Could you check a few things on this model? Use its own coordinates, in mm. A direction names the side the tool comes from. Round coordinates to 2 decimals unless told otherwise and drop trailing zeros. Write each loop counter-clockwise with the first axis right and the second up, starting at its lowest first coordinate (ties: lowest second). Pieces come first, ordered by that corner, then holes. Notation, with made-up numbers: (60, 31.5) -> (91, 31.5) arc R32 cw to (91, 68.5) -> close; hole circle Ø8 at (45.25, 64). An arc over 180 degrees is marked (long way). Answer in a Markdown table with one row per item.
from build123d import *

# Parameters (mm, degrees)
SKETCH_W      = 320
SKETCH_H      = 350
PAD_DEPTH     = 590
POCKET_DEPTH  = 50
SKETCH002_W   = 312.833359
SKETCH002_H   = 173.796318
SKETCH002_W_2 = 309.6734
SKETCH002_H_2 = 165.896453
PAD001_DEPTH  = 10
SKETCH003_W   = 329.541511
SKETCH003_H   = 368.861823
PAD002_DEPTH  = 50


with BuildPart() as part:
    # Sketch → Pad (new body)
    with BuildSketch(Plane.XZ):
        with Locations((160, 175)):
            Rectangle(SKETCH_W, SKETCH_H)
    extrude(amount=PAD_DEPTH)

    # Sketch001 (on Face6 of Pad) → Pocket (cut)
    with BuildSketch(Plane.XZ.offset(590)):
        Polygon((-35.069702, 294.049438), (-35.069702, 61.386997), (59.508472, 61.386997), (59.508472, -35.082802), (254.339645, -35.082802), (254.339645, 61.386997), (365.941986, 61.386997), (365.941986, 294.049438), (254.339645, 294.049438), (254.339645, 365.928894), (59.508472, 365.928894), (59.508472, 294.049438), align=None)
    extrude(amount=-POCKET_DEPTH, mode=Mode.SUBTRACT)

    # Sketch002 (on Face9 of Pocket) → Pad001 (join)
    with BuildSketch(Plane(origin=(0, 0, 0), x_dir=(0, 0, -1), z_dir=(-1, 0, 0))):
        with Locations((-177.158851, 160.656223)):
            Rectangle(SKETCH002_W, SKETCH002_H)
        with Locations((-177.158844, 363.681931)):
            Rectangle(SKETCH002_W_2, SKETCH002_H_2)
    extrude(amount=PAD001_DEPTH)

    # Sketch003 (on Face2 of Pad001) → Pad002 (join)
    with BuildSketch(Plane(origin=(0, 0, 0), x_dir=(1, 0, 0), z_dir=(0, 1, 0))):
        with Locations((159.986142, -175.059994)):
            Rectangle(SKETCH003_W, SKETCH003_H)
    extrude(amount=-PAD002_DEPTH)


solid = part.part
1) For pin 1 (1.5 mm diameter, centred on y = -383, z = 81.5, fed in from +X); pin 2 (25 mm diameter, centred on y = -36, z = 192, fed in from -X); pin 3 (8 mm diameter, centred on x = -5.5, y = -182, fed in from -Z), each with a flat end and sliding along its axis, tell me the tip position at first contact or that it passes through.
Findings:
| item | result |
|---|---|
| pin 1 | stops at x = 320 |
| pin 2 | stops at x = -4.78 |
| pin 3 | stops at z = 20.74 |
2) Please list where these lines run through material, in increasing order: line 1 (X direction, y = -143, z = 146); line 2 (Y direction, x = 159, z = 128); line 3 (Z direction, x = 134.5, y = -183).
Findings:
| item | result |
|---|---|
| line 1 | x = -10 to 320 |
| line 2 | y = -540 to 0 |
| line 3 | z = 0 to 350 |
3) Imagine slicing it at C-C, the plane x = 34. Please give me the cut outline in (y, z), plus the area to 3 significant figures.
Findings:
| item | result |
|---|---|
| outline | (-590, 0) -> (-50, 0) -> (-50, -9.37) -> (0, -9.37) -> (0, 359.49) -> (-50, 359.49) -> (-50, 350) -> (-590, 350) -> (-590, 294.05) -> (-540, 294.05) -> (-540, 61.39) -> (-590, 61.39) -> close |
| area | 196,000 mm^2 |
4) Thinking about a two-plate mould opening in Y: for faces 6 (the face through (29, -590, 31)), 7 (the face through (0, -479, 161)), 8 (the face through (158, -316, 0)), which applies, +Y half, -Y half, draft (parallel to the pull), parting line (faces both ways), or undercut?
Findings:
| item | result |
|---|---|
| face 6 | -Y half |
| face 7 | undercut |
| face 8 | draft |
5) Imagine slicing it at B-B, the plane y = -289. Please give me the cut outline in (x, z).
Findings:
| item | result |
|---|---|
| outline | (-10, 22.32) -> (0, 22.32) -> (0, 0) -> (320, 0) -> (320, 350) -> (0, 350) -> (0, 332) -> (-10, 332) -> close |
6) Imagine slicing it at A-A, the plane z = 275. Please give me the cut outline in (x, y), plus the area to 3 significant figures.
Findings:
| item | result |
|---|---|
| outline | (-10, -446.63) -> (0, -446.63) -> (0, -540) -> (320, -540) -> (320, -50) -> (324.76, -50) -> (324.76, 0) -> (-4.78, 0) -> (-4.78, -50) -> (0, -50) -> (0, -73.76) -> (-10, -73.76) -> (-10, -247.55) -> (0, -247.55) -> (0, -280.73) -> (-10, -280.73) -> close |
| area | 177,000 mm^2 |
7) For faces 1 (the face through (158, -25, -9.371)), 2 (the face through (30, -565, 294.049)), 3 (the face through (59.508, -565, 322)), 4 (the face through (320, -316, 173)), 5 (the face through (-4.785, -25, 178)), which set-ups out of +Z, -Z, +X, -X, +Y, -Y let a thin tool reach every point of the face, with its end or its side?
Findings:
| item | result |
|---|---|
| face 1 | -Z, +X, -X, +Y, -Y |
| face 2 | +X, -X, -Y |
| face 3 | +Z, -Z, -Y |
| face 4 | +Z, -Z, +X, -Y |
| face 5 | +Z, -Z, -X, +Y |
8) Imagine slicing it at D-D, the plane y = -142. Please give me the cut outline in (x, z), plus the area to 3 significant figures.
Findings:
| item | result |
|---|---|
| outline | (-10, 20.74) -> (0, 20.74) -> (0, 0) -> (320, 0) -> (320, 350) -> (0, 350) -> (0, 333.58) -> (-10, 333.58) -> close |
| area | 115,000 mm^2 |
